Read the model definition and answer for the solid it produces. Units are mm, in the model's axes. Give positions to 0.01 mm unless a question says otherwise; leave off trailing zeros. Write each loop counter-clockwise with the first axis right and the second up, starting at its lowest first coordinate (ties: lowest second). Pieces come first, ordered by that corner, then holes.
```python
from build123d import *

# Parameters (mm, degrees)
SKETCH1_W                = 215.9
SKETCH1_H                = 12.75
SKETCH1_R                = 1.55
BASE_FLANGE1_DEPTH       = 0.86
FILLET1_R                = 6
M3_CLEARANCE_HOLE1_D     = 3.4
M3_CLEARANCE_HOLE1_DEPTH = 1.29
M3_CLEARANCE_HOLE1_TIP   = 1.021463052
M3_CLEARANCE_HOLE2_D     = 3.4
M3_CLEARANCE_HOLE2_DEPTH = 1.29
M3_CLEARANCE_HOLE2_TIP   = 1.021463052
SKETCH14_R               = 1.55
CUT_EXTRUDE1_DEPTH       = 82


# Sheet-metal steps are written as plain solids
with BuildPart() as part:
    # Sketch1 → Base-Flange1 (new body)
    with BuildSketch(Plane(origin=(0, 0, 0), x_dir=(1, 0, 0), z_dir=(0, 1, 0))):
        Rectangle(SKETCH1_W, SKETCH1_H)
        with Locations(Location((-101.6, 0, 0), (0, 0, 270))):
            Circle(SKETCH1_R, mode=Mode.SUBTRACT)
    extrude(amount=-BASE_FLANGE1_DEPTH)

    # Fillet1
    fillet1_edges = [part.edges().sort_by_distance(p)[0] for p in [
        (-107.95, -0.43, -6.375),
        (107.95, -0.43, -6.375),
        (107.95, -0.43, 6.375),
        (-107.95, -0.43, 6.375),
    ]]
    fillet(fillet1_edges, radius=FILLET1_R)

    # M3 Clearance Hole1
    with Locations(Plane(origin=(0, 0, 0), x_dir=(1, 0, 0), z_dir=(0, 1, 0))):
        with Locations((-80.011608413, 0.075207541), (-24.131608413, 0.075207541), (80.01, 0), (24.13, 0)):
            Hole(M3_CLEARANCE_HOLE1_D / 2, depth=M3_CLEARANCE_HOLE1_DEPTH)
            with Locations((0, 0, -(M3_CLEARANCE_HOLE1_DEPTH + M3_CLEARANCE_HOLE1_TIP / 2))):  # 118° drill point
                Cone(0, M3_CLEARANCE_HOLE1_D / 2, M3_CLEARANCE_HOLE1_TIP, mode=Mode.SUBTRACT)

    # M3 Clearance Hole2
    with Locations(Plane(origin=(0, 0, 0), x_dir=(1, 0, 0), z_dir=(0, 1, 0))):
        with Locations((0, 0), (-53.975, 0), (53.975, 0)):
            Hole(M3_CLEARANCE_HOLE2_D / 2, depth=M3_CLEARANCE_HOLE2_DEPTH)
            with Locations((0, 0, -(M3_CLEARANCE_HOLE2_DEPTH + M3_CLEARANCE_HOLE2_TIP / 2))):  # 118° drill point
                Cone(0, M3_CLEARANCE_HOLE2_D / 2, M3_CLEARANCE_HOLE2_TIP, mode=Mode.SUBTRACT)

    # Sketch14 → Cut-Extrude1 (cut)
    with BuildSketch(Plane(origin=(0, 0, 0), x_dir=(1, 0, 0), z_dir=(0, 1, 0))):
        with Locations(Location((101.601385273, -0.242368773, 0), (0, 0, 270))):
            Circle(SKETCH14_R)
    extrude(amount=-CUT_EXTRUDE1_DEPTH, mode=Mode.SUBTRACT)


solid = part.part
```
Item 1: This flat-tipped pin is pushed along its axis until it touches: pin 1 Ø3 at (x, z) = (53.975, 0) entering from -Y. Where does it stop, or does it pass through?
Result set:
pin 1: passes through
Item 2: Section A-A (y = -0.6) is taken. Give the number of separate pieces and of enclosed holes in the cut face, and give its area (3 significant figures).
Result set:
separate pieces: 1
enclosed holes: 9
area: 2,640 mm2
Item 3: Find the intervals of material crossed by line 1 along Z through (x, y) = (80.01, -0.65) (3 decimals); line 2 along Z through (x, y) = (-101.6, -0.35) (3 decimals); line 3 along X through (y, z) = (-0.1, 5.5), in increasing order.
Result set:
line 1: z = -6.375 to -1.7, 1.7 to 6.375
line 2: z = -6.375 to -1.55, 1.55 to 6.375
line 3: x = -105.07 to 105.07
Item 4: Determine the mould class of faces 1 (the cylindrical face through (-25.75, -0.44, -0.59)), 2 (the flat face through (-2, -0.86, -2)), 3 (the cylindrical face through (106.15, -0.44, -4.66)) for opening direction X: pulls with the +X half, pulls with the -X half, needs draft (parallel to the pull), parting line crosses it, or undercut.
Result set:
face 1: undercut
face 2: needs draft
face 3: pulls with the +X half
Item 5: Section B-B (z = -4.5) is taken. Write down the section's boundary in (x, y).
Result set:
outline: (-106.31, -0.86) - (106.31, -0.86) - (106.31, 0) - (-106.31, 0) - close
